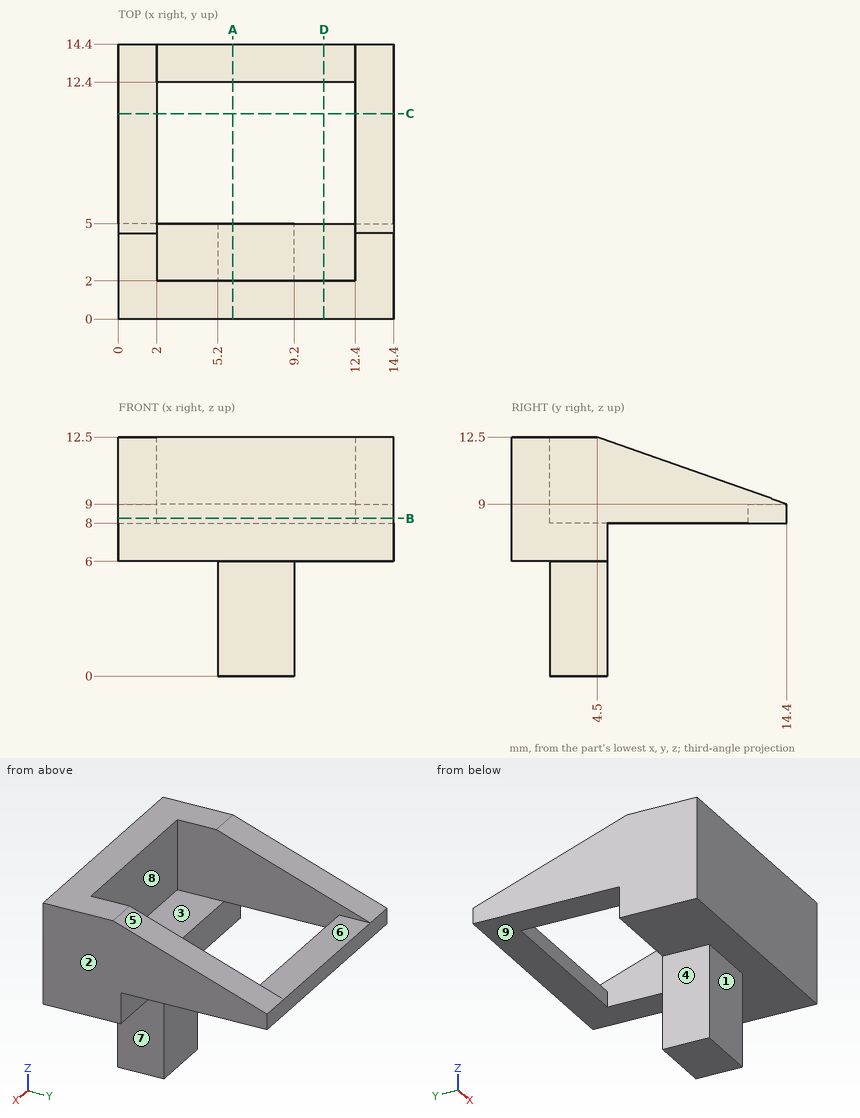
Answer from the drawing. Dimensions are ordinates in mm from the lowest x, y and z of the part. A direction names the side the tool comes from. Give positions to 0.01 mm unless a question says otherwise; leave off trailing zeros. Order: outer loops, then holes, each group sorted by start corner. A loop starts at its lowest first (then second) coordinate and runs counter-clockwise, first axis right, second up. Notation, with made-up numbers: (27, -33.75) -> (63, -33.75) arc R29 cw to (63, 5.25) -> close; hole circle Ø10 at (13.5, -28.5). An arc over 180 degrees is marked (long way). One line per item, written item: value. Start each with the question number.
(1) For a pull along X with two mould halves and no side action, classify the marked faces 1, 2, 3 and 4 as released by +X, released by -X, zero draft, split by the parting line, or undercut.
(2) The part is cut by section B-B (z = 8.25). Determine the outline of the cut face in (x, y).
(3) The part is cut by section D-D (x = 10.75). Determine the outline of the cut face in (y, z), and give its area (3 significant figures).
(4) Straight lines are drawn through the part: L1, parallel to Y at x = 8.25, z = 8.75; L2, parallel to Y at x = 8.75, z = 2. For each, find the intervals that lie inside material, in ascending order.
(5) A tool of negligible diameter and unlimited length cuts with its end or side. For the marked faces 5, 6, 7, 8 and 9, from which of +Z, -Z, +X, -X, +Y, -Y can it reach the whole face along a straight path? Write none if from no direction.
(6) Flat-ended cylindrical pins translate along their axes: P1, Ø3, axis at y = 11, z = 6, coming from the -X side; P2, Ø6, axis at x = 5.5, z = 2, coming from the -Y side; P3, Ø1, axis at x = 5, y = 13, coming from the +Z side; P4, Ø2.5, axis at y = 3, z = 1.5, coming from the -X side. Find the tip coordinate at first contact, or state that the pin passes through.
(7) The part is cut by section C-C (y = 10.75). Determine the outline of the cut face in (x, z).
(8) The part is cut by section A-A (x = 6). Determine the outline of the cut face in (y, z), and give its area (3 significant figures).
Taken from the geometry:
1. face 1: zero draft
1. face 2: released by +X
1. face 3: undercut
1. face 4: released by -X
2. outline: (0, 0) -> (14.4, 0) -> (14.4, 14.4) -> (0, 14.4) -> close; hole (2, 2) -> (12.4, 2) -> (12.4, 12.4) -> (2, 12.4) -> close
3. outline: (0, 6) -> (5, 6) -> (5, 8) -> (2, 8) -> (2, 12.5) -> (0, 12.5) -> close; (12.4, 8) -> (14.4, 8) -> (14.4, 9) -> (12.4, 9) -> close
3. area: 21.0 mm^2
4. L1: 0 to 2, 12.4 to 14.4
4. L2: 2 to 5
5. face 5: +Z, +X, -X, +Y
5. face 6: +Z, +Y
5. face 7: -Z, +X, +Y, -Y
5. face 8: +Z
5. face 9: -Z, +X, -X, +Y
6. P1: through
6. P2: y = 2
6. P3: z = 9
6. P4: x = 5.2
7. outline: (0, 8) -> (2, 8) -> (2, 10.29) -> (0, 10.29) -> close; (12.4, 8) -> (14.4, 8) -> (14.4, 10.29) -> (12.4, 10.29) -> close
8. outline: (0, 6) -> (2, 6) -> (2, 0) -> (5, 0) -> (5, 8) -> (2, 8) -> (2, 12.5) -> (0, 12.5) -> close; (12.4, 8) -> (14.4, 8) -> (14.4, 9) -> (12.4, 9) -> close
8. area: 39.0 mm^2
